from build123d import *

# Parameters (mm, degrees)
CYLINDER009_R     = 0.7
CYLINDER009_DEPTH = 16
BOX010_W          = 12.25
BOX010_H          = 10
BOX010_DEPTH      = 10
BOX009_W          = 12.25
BOX009_H          = 23.78
BOX009_DEPTH      = 22.68
BOX011_W          = 24.3
BOX011_H          = 21
BOX011_DEPTH      = 30
CYLINDER012_R     = 3
CYLINDER012_DEPTH = 1
CYLINDER013_R     = 2.4
CYLINDER013_DEPTH = 8
CYLINDER011_R     = 3
CYLINDER011_DEPTH = 1
ARRAY_X_COUNT     = 2
ARRAY_X_PITCH     = 32
BOX012_W          = 40
BOX012_H          = 8
BOX012_DEPTH      = 8


with BuildPart() as cylinder009:
    # Cylinder009 → Cylinder009 (new body)
    with BuildSketch(Plane(origin=(6, 22, 25), x_dir=(1, 0, 0), z_dir=(0, -1, 0))):
        Circle(CYLINDER009_R)
    extrude(amount=CYLINDER009_DEPTH)


with BuildPart() as cube006:
    # Box010 → Box010 (new body)
    with BuildSketch(Plane(origin=(0, -3.25, 22), x_dir=(1, 0, 0), z_dir=(0, 0, 1))):
        with Locations((6.125, 5)):
            Rectangle(BOX010_W, BOX010_H)
    extrude(amount=BOX010_DEPTH)


with BuildPart() as servo004:
    # Box009 → Box009 (new body)
    with BuildSketch(Plane(origin=(0, -1, 0), x_dir=(1, 0, 0), z_dir=(0, 0, 1))):
        with Locations((6.125, 11.89)):
            Rectangle(BOX009_W, BOX009_H)
    extrude(amount=BOX009_DEPTH)

    # Fusion007: union Cube006
    add(cube006.part)


with BuildPart() as fusion008:
    # Fusion008 base: copy of Cube006
    add(cube006.part)

    # Fusion008: union servo004
    add(servo004.part)


with BuildPart() as box:
    # Box011 → Box011 (new body)
    with BuildSketch(Plane(origin=(-6, 0, 0), x_dir=(1, 0, 0), z_dir=(0, 0, 1))):
        with Locations((12.15, 10.5)):
            Rectangle(BOX011_W, BOX011_H)
    extrude(amount=BOX011_DEPTH)

    # Cut006: cut Fusion008
    add(fusion008.part, mode=Mode.SUBTRACT)

    # Cut007: cut Cylinder009
    add(cylinder009.part, mode=Mode.SUBTRACT)


with BuildPart() as box_1:
    # Cut007 placement: moved
    add(box.part.moved(Location((9.85, -17, 8))))


with BuildPart() as cylinder012:
    # Cylinder012 → Cylinder012 (new body)
    with BuildSketch(Plane.XY.offset(7)):
        Circle(CYLINDER012_R)
    extrude(amount=CYLINDER012_DEPTH)


with BuildPart() as cylinder013:
    # Cylinder013 → Cylinder013 (new body)
    with BuildSketch(Plane.XY):
        Circle(CYLINDER013_R)
    extrude(amount=CYLINDER013_DEPTH)


with BuildPart() as array:
    # Cylinder011 → Cylinder011 (new body)
    with BuildSketch(Plane.XY):
        Circle(CYLINDER011_R)
    extrude(amount=CYLINDER011_DEPTH)

    # Fusion009: union Cylinder012, Cylinder013
    add(cylinder012.part)
    add(cylinder013.part)

    # Array X: Array ×2


with BuildPart() as array_1:
    add(array.part)
    with Locations(*[(i * ARRAY_X_PITCH, 0, 0) for i in range(1, ARRAY_X_COUNT)]):
        add(array.part)


with BuildPart() as fusion010:
    # Box012 → Box012 (new body)
    with BuildSketch(Plane(origin=(-4, -4, 0), x_dir=(1, 0, 0), z_dir=(0, 0, 1))):
        with Locations((20, 4)):
            Rectangle(BOX012_W, BOX012_H)
    extrude(amount=BOX012_DEPTH)

    # Cut008: cut Array
    add(array_1.part, mode=Mode.SUBTRACT)

    # Fusion010: union box
    add(box_1.part)


solid = fusion010.part
Input: part model. Units: mm. Frame: model coordinates. A direction names the side the tool comes from. Coordinates: 2 decimals unless noted, no trailing zeros. Loops run counter-clockwise (first coordinate to the right, second up) from the corner with the lowest first, then second, coordinate; pieces in that order, holes last. Notation, with made-up numbers: (14.25, 7.5) -> (36.25, 7.5) arc R35 cw to (36.25, 45.5) -> close; hole circle Ø2 at (64, 49). An arc over 180 degrees is marked (long way). One line per item, written item: value.
(1) Cut plane C-C (z = 33). Output: boundary loops of the cut face in (x, y).
Answer below:
outline: (3.85, -17) -> (9.85, -17) -> (9.85, -10.25) -> (15.15, -10.25) -> (15.15, 4) -> (3.85, 4) -> close; (16.55, -10.25) -> (22.1, -10.25) -> (22.1, -17) -> (28.15, -17) -> (28.15, 4) -> (16.55, 4) -> close
(2) Cut plane B-B (y = -13.5). Output: boundary loops of the cut face in (x, z), then the cut area to 4 significant figures.
Answer below:
outline: (3.85, 8) -> (9.85, 8) -> (9.85, 38) -> (3.85, 38) -> close; (22.1, 8) -> (28.15, 8) -> (28.15, 38) -> (22.1, 38) -> close
area: 361.5 mm2
(3) Draft query along Z for faces 5 (the face through (35, 2, 8)), 6 (the face through (3.85, -7, 23)), 7 (the face through (9.85, -7, 19)). Return one class per face: pulls with the +Z half, pulls with the -Z half, needs draft (parallel to the pull), parting line crosses it, or undercut.
Answer below:
face 5: pulls with the +Z half
face 6: needs draft
face 7: undercut
(4) Cut plane D-D (y = 0). Give the number of separate pieces and of enclosed holes in the cut face, then the cut area to 3 significant figures.
Answer below:
separate pieces: 3
enclosed holes: 2
area: 688 mm2
(5) Cut plane A-A (x = 18.5). Output: boundary loops of the cut face in (y, z).
Answer below:
outline: (-10.25, 30.68) -> (4, 30.68) -> (4, 38) -> (-10.25, 38) -> close; (-4, 0) -> (4, 0) -> (4, 8) -> (-4, 8) -> close
(6) Set-up query: faces 1 (the face through (16, 0, 8)), 2 (the face through (-3, -2, 8)), 3 (the face through (29, 0.1, 7.5)), 4 (the face through (28.15, -7, 23)). Return all of +Z, -Z, +X, -X, +Y, -Y with unobstructed straight access to the full face (end or side cutting, diameter ignored); none if empty.
Answer below:
face 1: +Y, -Y
face 2: +Z, -X, +Y, -Y
face 3: +Z
face 4: +Z, +X, +Y, -Y
(7) Pin query (flat end, axial travel): pin 1 Ø7.5 at (x, y) = (32, 0) entering from +Z; pin 2 Ø4 at (y, z) = (-10.5, 23) entering from -X; pin 3 Ø5.5 at (x, y) = (0, 0) entering from -Z; pin 4 Ø3 at (x, y) = (30.5, -11) entering from -Z. Return the tip coordinate at first contact, or that it passes through.
Answer below:
pin 1: stops at z = 8
pin 2: stops at x = 3.85
pin 3: stops at z = 1
pin 4: passes through
(8) Ray query, line 1 along X through (y, z) = (0, 4.3); line 2 along X through (y, z) = (-4, 20.5); line 3 along Y through (x, z) = (32, 2.6). Return the intervals inside material, ascending.
Answer below:
line 1: x = -4 to -2.4, 2.4 to 29.6, 34.4 to 36
line 2: x = 3.85 to 9.85, 22.1 to 28.15
line 3: y = -4 to -2.4, 2.4 to 4
